Part print with two shaded views. Sizes in mm from the minimum x, y, z corner. A direction names the side the tool comes from. Round coordinates to 2 decimals unless told otherwise and drop trailing zeros. Loops run counter-clockwise (first coordinate to the right, second up) from the corner with the lowest first, then second, coordinate; pieces in that order, holes last.
(1) Cut at C-C on x = 4. Count the separate pieces of the cut face and the enclosed holes in it.
(2) Tool access for the marked faces 1 and 2: list every direction of +Z, -Z, +X, -X, +Y, -Y with a clear straight run to the whole face (end or side of a thin tool).
(3) Probe probe 1 along Z at (x, y) = (3, 3.3) (1 decimal); probe 2 along X at (y, z) = (0.6, 17); probe 3 along Z at (x, y) = (4.25, 4.7) (1 decimal). List the from-to ranges inside material, lowest first.
(4) Cut at B-B on y = 3.3. List the corners of the cut face in (x, z).
(5) Flat gauge pins, fed straight in: pin 1 (2.5 mm diameter, centred on x = 3.5, z = 6, fed in from -Y); pin 2 (1 mm diameter, centred on x = 4.5, y = 3, fed in from -Z); pin 3 (3.5 mm diameter, centred on x = 3.5, z = 17, fed in from +Y). Where does each tip first touch, or does it go through?
(6) Mould opens along X. For the marked faces 3, 4 and 5 say: +X half, -X half, draft (parallel to the pull), parting line (faces both ways), or undercut.
(7) Cut at D-D on x = 0.75. List the corners of the cut face in (y, z) (1 decimal), then the cut area to 3 significant figures.
(8) Cut at A-A on z = 17. List the corners of the cut face in (x, y).
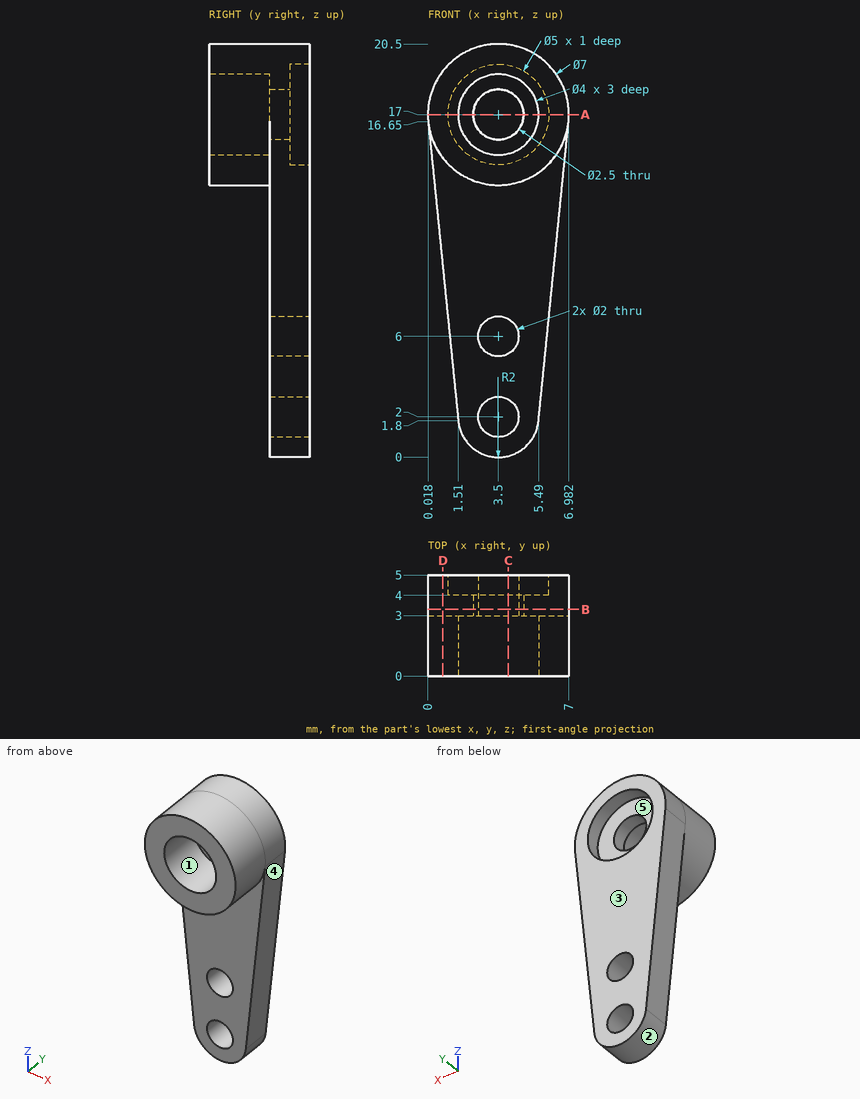
Final values:
1. separate pieces: 4
1. enclosed holes: 0
2. face 1: -Y
2. face 2: -Z, +Y, -Y
3. probe 1: z = 0.1 to 1.1, 2.9 to 5.1, 6.9 to 15.9, 18.1 to 20.5
3. probe 2: x = 0 to 1.5, 5.5 to 7
3. probe 3: z = 0.1 to 1.3, 2.7 to 5.3, 6.7 to 14.6, 19.4 to 20.4
4. outline: (0.02, 16.65) - (1.51, 1.8) arc R2 ccw to (5.49, 1.8) - (6.98, 16.65) arc R3.5 ccw (long way) to start; hole circle Ø2.5 at (3.5, 17); hole circle Ø2 at (3.5, 2); hole circle Ø2 at (3.5, 6)
5. pin 1: stops at y = 3
5. pin 2: stops at z = 0.06
5. pin 3: stops at y = 4
6. face 3: draft
6. face 4: +X half
6. face 5: undercut
7. outline: (0, 14.8) - (3, 14.8) - (3, 9.4) - (5, 9.4) - (5, 19.2) - (0, 19.2) - close
7. area: 32.6 mm2
8. outline: (0, 0) - (1.5, 0) - (1.5, 3) - (2.25, 3) - (2.25, 4) - (1, 4) - (1, 5) - (0, 5) - close; (4.75, 3) - (5.5, 3) - (5.5, 0) - (7, 0) - (7, 5) - (6, 5) - (6, 4) - (4.75, 4) - close
